from build123d import *

# Parameters (mm, degrees)
SKETCH_1_W               = 42
SKETCH_1_H               = 25
EXTRUDE_1_DEPTH          = 12
SKETCH_3_W               = 10
SKETCH_3_H               = 21
CUT_EXTRUDE_1_DEPTH      = 41
SKETCH_4_W               = 5
SKETCH_4_H               = 10
CUT_EXTRUDE_2_DEPTH      = 10
SKETCH_5_W               = 12
SKETCH_5_H               = 4
CUT_EXTRUDE_3_DEPTH      = 10
CUT_EXTRUDE_4_DEPTH      = 10
CUT_EXTRUDE_4_DEPTH_BACK = 10
SKETCH_6_R               = 1
FILLET_1_R               = 1


with BuildPart() as part:
    # Sketch 1 → Extrude 1 (new body)
    with BuildSketch(Plane.XY):
        Rectangle(SKETCH_1_W, SKETCH_1_H)
    extrude(amount=EXTRUDE_1_DEPTH)

    # Sketch 3 → Cut-Extrude 1 (cut)
    with BuildSketch(Plane(origin=(21, 0, 0), x_dir=(0, 0, -1), z_dir=(1, 0, 0))):
        with Locations((-6, 0)):
            Rectangle(SKETCH_3_W, SKETCH_3_H)
    extrude(amount=-CUT_EXTRUDE_1_DEPTH, mode=Mode.SUBTRACT)

    # Sketch 4 → Cut-Extrude 2 (cut)
    with BuildSketch(Plane(origin=(-20, 0, 0), x_dir=(0, 0, -1), z_dir=(1, 0, 0))):
        with Locations((-8.5, 0)):
            Rectangle(SKETCH_4_W, SKETCH_4_H)
    extrude(amount=-CUT_EXTRUDE_2_DEPTH, mode=Mode.SUBTRACT)

    # Sketch 5 → Cut-Extrude 3 (cut)
    with BuildSketch(Plane.XY.offset(12)):
        with Locations((15, 8.5)):
            Rectangle(SKETCH_5_W, SKETCH_5_H)
        with Locations((15, -8.5)):
            Rectangle(SKETCH_5_W, SKETCH_5_H)
    extrude(amount=-CUT_EXTRUDE_3_DEPTH, mode=Mode.SUBTRACT)

    # Sketch 6 → Cut-Extrude 4 (cut, two sides: drawn at the far end of the back side and taken through both)
    with BuildSketch(Plane.XY.offset(12).offset(-CUT_EXTRUDE_4_DEPTH_BACK)):
        with Locations(Location((-15, 7, 0), (0, 0, 180))):
            Circle(SKETCH_6_R)
        with Locations(Location((-15, -7, 0), (0, 0, 180))):
            Circle(SKETCH_6_R)
    extrude(amount=CUT_EXTRUDE_4_DEPTH + CUT_EXTRUDE_4_DEPTH_BACK, mode=Mode.SUBTRACT)

    # Fillet 1
    fillet_1_edges = [part.edges().sort_by_distance(p)[0] for p in [
        (0, -12.5, 12),
        (0, 12.5, 12),
        (0, -12.5, 0),
        (0, 12.5, 0),
    ]]
    fillet(fillet_1_edges, radius=FILLET_1_R)


solid = part.part
Verification items for the finished model (mm, model axes). A direction names the side the tool comes from. Give positions to 0.01 mm unless a question says otherwise; leave off trailing zeros. Write each loop counter-clockwise with the first axis right and the second up, starting at its lowest first coordinate (ties: lowest second). Pieces come first, ordered by that corner, then holes. Notation, with made-up numbers: (-28.75, -25.75) - (-9.75, -25.75) arc R7 ccw to (-9.75, -12.75) - close; hole circle Ø6 at (88, 86.5). An arc over 180 degrees is marked (long way). Answer as CSV lines item,"result". Start each with the question number.
1. Thickness scan on line 1 (Y direction, x = -19, z = 10.5); line 2 (Z direction, x = -11.5, y = -6.5); line 3 (Y direction, x = -15, z = 11.6). Record the ranges inside material, lowest first.
2. Depth check by flat-ended pin: pin 1 (1 mm diameter, centred on y = 6, z = 2, fed in from +X); pin 2 (0.5 mm diameter, centred on x = 16, z = 11.5, fed in from +Y); pin 3 (1.1 mm diameter, centred on y = 9, z = 11.5, fed in from +X). Enter the tip coordinate at first touch or a pass-through.
3. Sectioned sample at B-B (z = 9.25). Record the boundary of the cut face in (x, y), then the cut area to 3 significant figures.
4. Sectioned sample at D-D (z = 3.5). Record the boundary of the cut face in (x, y), then the cut area to 3 significant figures.
5. Draft check along Z on faces 6 (the face through (0.294, 12.199, 11.715)), 7 (the face through (21, -0.1, 0.6)), 8 (the face through (-20.5, -5, 8.5)). Enter one of: pulls with the +Z half, pulls with the -Z half, needs draft (parallel to the pull), parting line crosses it, or undercut.
6. Sectioned sample at A-A (y = -7). Record the boundary of the cut face in (x, z).
7. Sectioned sample at C-C (x = 3.5). Record the boundary of the cut face in (y, z).
8. Set-up check for faces 1 (the face through (-15.954, 6.7, 11.493)), 2 (the face through (0, -12.5, 6)), 3 (the face through (9, -8.5, 11.5)), 4 (the face through (-4, 0, 11)), 5 (the face through (-20.5, -0.1, 6)): record each of +Z, -Z, +X, -X, +Y, -Y from which the full face is reachable in a straight line by a thin tool's end or side.
Derived:
1,line 1,"-12.5 to -10.5, 10.5 to 12.5"
1,line 2,"0 to 1, 11 to 12"
1,line 3,"-12.3 to -8, -6 to 6, 8 to 12.3"
2,pin 1,"x = -20"
2,pin 2,"y = 12.47"
2,pin 3,"x = 9"
3,outline,"(-21, -12.5) - (21, -12.5) - (21, -10.5) - (-20, -10.5) - (-20, -5) - (-21, -5) - close; (-21, 5) - (-20, 5) - (-20, 10.5) - (21, 10.5) - (21, 12.5) - (-21, 12.5) - close"
3,area,"179 mm²"
4,outline,"(-21, -12.5) - (21, -12.5) - (21, -10.5) - (-20, -10.5) - (-20, 10.5) - (21, 10.5) - (21, 12.5) - (-21, 12.5) - close"
4,area,"189 mm²"
5,face 6,"pulls with the +Z half"
5,face 7,"needs draft"
5,face 8,"undercut"
6,outline,"(-21, 0) - (21, 0) - (21, 1) - (-20, 1) - (-20, 11) - (-16, 11) - (-16, 12) - (-21, 12) - close; (-14, 11) - (9, 11) - (9, 12) - (-14, 12) - close"
7,outline,"(-12.5, 1) arc R1 ccw to (-11.5, 0) - (11.5, 0) arc R1 ccw to (12.5, 1) - (12.5, 11) arc R1 ccw to (11.5, 12) - (-11.5, 12) arc R1 ccw to (-12.5, 11) - close; hole (-10.5, 1) - (10.5, 1) - (10.5, 11) - (-10.5, 11) - close"
8,face 1,"+Z"
8,face 2,"+Z, -Z, +X, -X, -Y"
8,face 3,"+Z, +X"
8,face 4,"+X"
8,face 5,"+X, -X"
